```python
from build123d import *

# Parameters (mm, degrees)
SKETCH1_W           = 25.4
SKETCH1_H           = 25.4
SKETCH1_W_2         = 23.6
SKETCH1_H_2         = 23.6
EXTRUDE_THIN1_DEPTH = 250
SKETCH2_R           = 4
CUT_EXTRUDE1_DEPTH  = 252.607730406
SKETCH3_R           = 3
SKETCH3_R_2         = 4
SKETCH3_R_3         = 5.1
CUT_EXTRUDE2_DEPTH  = 252.607730406


with BuildPart() as part:
    # Sketch1 → Extrude-Thin1 (new, symmetric)
    with BuildSketch(Plane.XY):
        Rectangle(SKETCH1_W, SKETCH1_H)
        Rectangle(SKETCH1_W_2, SKETCH1_H_2, mode=Mode.SUBTRACT)
    extrude(amount=EXTRUDE_THIN1_DEPTH, both=True)

    # Sketch2 → Cut-Extrude1 (cut, through all)
    with BuildSketch(Plane(origin=(12.7, 0, 0), x_dir=(0, 0, -1), z_dir=(1, 0, 0))):
        with Locations(Location((156.7, 0, 0), (0, 0, 90))):
            Circle(SKETCH2_R)
        with Locations(Location((230, 0, 0), (0, 0, 90))):
            Circle(SKETCH2_R)
        with Locations(Location((94.7, 0, 0), (0, 0, 90))):
            Circle(SKETCH2_R)
        with Locations(Location((-213.12, 0, 0), (0, 0, 90))):
            Circle(SKETCH2_R)
    extrude(amount=-CUT_EXTRUDE1_DEPTH, mode=Mode.SUBTRACT)

    # Sketch3 → Cut-Extrude2 (cut, through all)
    with BuildSketch(Plane.XZ.offset(12.7)):
        with Locations(Location((0, 239.8, 0), (0, 0, 270))):
            Circle(SKETCH3_R)
        with Locations(Location((0, -137.65, 0), (0, 0, 270))):
            Circle(SKETCH3_R_2)
        with Locations(Location((0, -193.35, 0), (0, 0, 270))):
            Circle(SKETCH3_R_3)
    extrude(amount=-CUT_EXTRUDE2_DEPTH, mode=Mode.SUBTRACT)


solid = part.part
```
Here's how the part is built. I have some questions about the finished solid (model axes, mm). A direction names the side the tool comes from. Round coordinates to 2 decimals unless told otherwise and drop trailing zeros. Order: outer loops, then holes, each group sorted by start corner. A loop starts at its lowest first (then second) coordinate and runs counter-clockwise, first axis right, second up. Notation, with made-up numbers: M 34,20 L 80,20 A18 ccw 80,35 Z; hole C -13,-0.75 d7. An arc over 180 degrees is marked long. Answer as CSV lines item,"result".
Item 1: Imagine slicing it at B-B on z = -193.35. List the corners of the cut face in (x, y) for me, and give its area (3 significant figures).
From the geometry:
outline,"M -12.7,-12.7 L -5.1,-12.7 L -5.1,-11.8 L -11.8,-11.8 L -11.8,11.8 L -5.1,11.8 L -5.1,12.7 L -12.7,12.7 Z; M 5.1,-12.7 L 12.7,-12.7 L 12.7,12.7 L 5.1,12.7 L 5.1,11.8 L 11.8,11.8 L 11.8,-11.8 L 5.1,-11.8 Z"
area,"69.8 mm2"
Item 2: For pin 1 (5 mm diameter, centred on y = 0, z = -156.7, fed in from +X), with a flat end and sliding along its axis, tell me the tip position at first contact or that it passes through.
From the geometry:
pin 1,"through"
Item 3: Which directions (+Z, -Z, +X, -X, +Y, -Y) give clear straight access to the entire face, cutting with the end or side of a thin tool? Please do faces 4 (the flat face through (0, 11.8, 4)), 5 (the cylindrical face through (-12.244, -0.867, 209.215)).
From the geometry:
face 4,"+Z, -Z"
face 5,"+X, -X"
Item 4: We'd pull the mould along Y, two halves only. Please class faces 1 (the cylindrical face through (0.176, -12.256, -133.654)), 2 (the flat face through (0, 12.7, 4)), 3 (the cylindrical face through (12.256, -0.867, 209.215)): +Y half, -Y half, draft (parallel to the pull), parting line (faces both ways), or undercut.
From the geometry:
face 1,"draft"
face 2,"+Y half"
face 3,"undercut"
Item 5: Imagine slicing it at A-A on z = 42.5. List the corners of the cut face in (x, y) for me, and give its area (3 significant figures).
From the geometry:
outline,"M -12.7,-12.7 L 12.7,-12.7 L 12.7,12.7 L -12.7,12.7 Z; hole M -11.8,-11.8 L 11.8,-11.8 L 11.8,11.8 L -11.8,11.8 Z"
area,"88.2 mm2"
Item 6: Imagine slicing it at C-C on y = 0. Give the number of separate pieces and of enclosed holes in the cut face, and give its area (3 significant figures).
From the geometry:
separate pieces,"10"
enclosed holes,"0"
area,"842 mm2"
Item 7: Please list where these lines run through material, in increasing order: L1, parallel to Z at x = -12.1, y = 0; L2, parallel to X at y = 10.75, z = -74. Write a range as [from, to].
From the geometry:
L1,"[-250, -234], [-226, -160.7], [-152.7, -98.7], [-90.7, 209.12], [217.12, 250]"
L2,"[-12.7, -11.8], [11.8, 12.7]"
